Input: dimensioned drawing with shaded views. Units: mm. Origin: part minimum x, y, z. A direction names the side the tool comes from. Coordinates: 2 decimals unless noted, no trailing zeros. Loops run counter-clockwise (first coordinate to the right, second up) from the corner with the lowest first, then second, coordinate; pieces in that order, holes last. Notation, with made-up numbers: (-1, -19.5) -> (53, -19.5) arc R20 cw to (53, -14.5) -> close; hole circle Ø7 at (1.25, 60.25). An arc over 180 degrees is marked (long way). Answer as CSV lines item,"result".
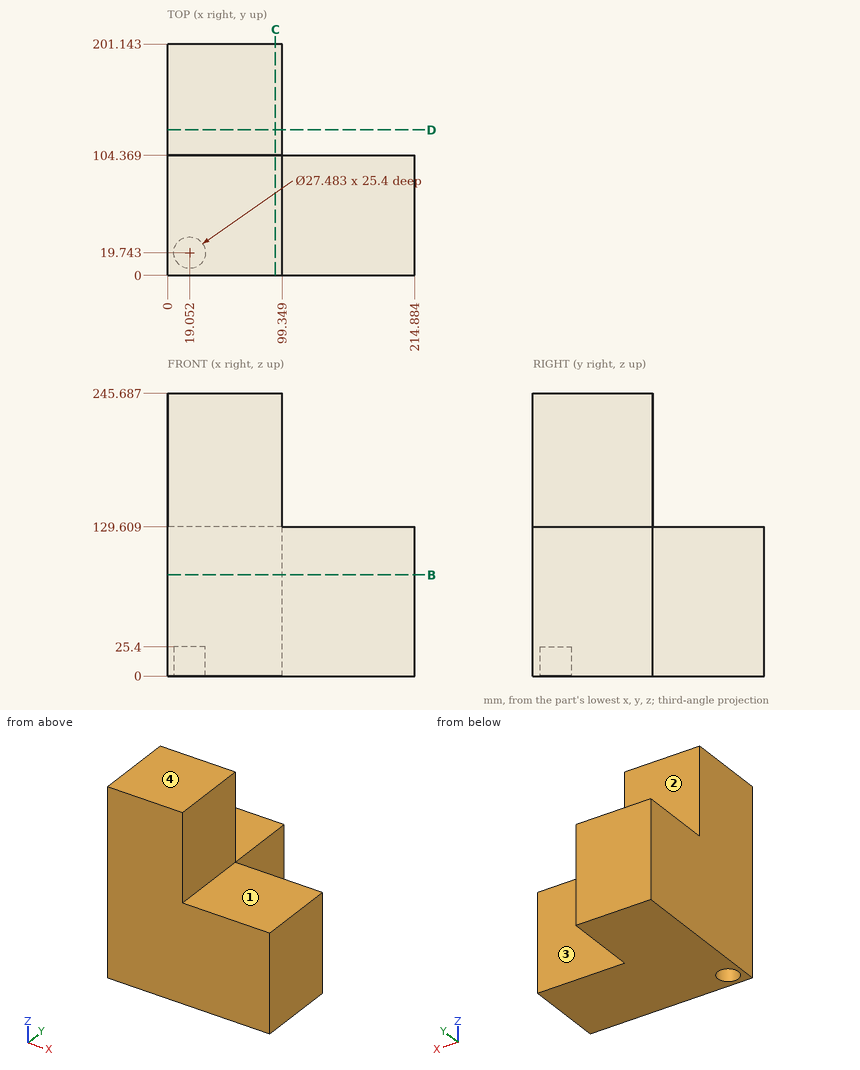
(1) Cut plane D-D (y = 126.5). Return the cut outline in (x, z), then the cut area to 3 significant figures.
Computed values:
outline,"(0, 0) -> (99.35, 0) -> (99.35, 129.61) -> (0, 129.61) -> close"
area,"12,900 mm^2"
(2) Cut plane C-C (x = 93.5). Return the cut outline in (y, z), then the cut area to 3 significant figures.
Computed values:
outline,"(0, 0) -> (201.14, 0) -> (201.14, 129.61) -> (104.37, 129.61) -> (104.37, 245.69) -> (0, 245.69) -> close"
area,"38,200 mm^2"
(3) Pin query (flat end, axial travel): pin 1 Ø12 at (x, z) = (172, 39.5) entering from +Y; pin 2 Ø8 at (x, z) = (166, 49.5) entering from -Y; pin 3 Ø16.5 at (x, y) = (19.05, 19.74) entering from -Z; pin 4 Ø4 at (x, y) = (152.5, 35.5) entering from +Z. Return the tip coordinate at first contact, or that it passes through.
Computed values:
pin 1,"y = 104.37"
pin 2,"y = 0"
pin 3,"z = 25.4"
pin 4,"z = 129.61"
(4) Cut plane B-B (z = 88). Return the cut outline in (x, y), then the cut area to 3 significant figures.
Computed values:
outline,"(0, 0) -> (214.88, 0) -> (214.88, 104.37) -> (99.35, 104.37) -> (99.35, 201.14) -> (0, 201.14) -> close"
area,"32,000 mm^2"
(5) Access query for the marked faces 1, 2, 3 and 4. Directions: +Z, -Z, +X, -X, +Y, -Y. A direction counts if a zero-diameter tool reaches every point of the face in a straight line with its end or side. Return the directions, or none.
Computed values:
face 1,"+Z, +X, +Y, -Y"
face 2,"+Z, +X, -X, +Y"
face 3,"+Z, -Z, +X, +Y"
face 4,"+Z, +X, -X, +Y, -Y"
(6) Material intervals for L1, parallel to Z at x = 175.5, y = 9; L2, parallel to Y at x = 102, z = 16.5; L3, parallel to X at y = 182, z = 63, sorted ascending. Write a range as [from, to].
Computed values:
L1,"[0, 129.61]"
L2,"[0, 104.37]"
L3,"[0, 99.35]"
